```python
from build123d import *

# Parameters (mm, degrees)
SKETCH1_R           = 3.5875
SKETCH1_R_2         = 1.5875
BOSS_EXTRUDE1_DEPTH = 10
SKETCH2_R           = 1.5875
BOSS_EXTRUDE2_DEPTH = 10
BOSS_EXTRUDE3_REACH = 7.279


with BuildPart() as part:
    # Sketch1 → Boss-Extrude1 (new body)
    with BuildSketch(Plane.XY):
        Circle(SKETCH1_R)
        Circle(SKETCH1_R_2, mode=Mode.SUBTRACT)
    extrude(amount=BOSS_EXTRUDE1_DEPTH)

    # Sketch2 → Boss-Extrude2 (add)
    with BuildSketch(Plane(origin=(0, -1.69195383, 0), x_dir=(1, 0, 0), z_dir=(0, 1, 0))):
        with BuildLine():
            Line((-3.5875, -5), (-3.5875, -10))
            Line((-3.5875, -10), (3.5875, -10))
            Line((3.5875, -10), (3.5875, -5))
            ThreePointArc((3.5875, -5), (0, -1.4125), (-3.5875, -5))
        make_face()
        with Locations((0, -5)):
            Circle(SKETCH2_R, mode=Mode.SUBTRACT)
    extrude(amount=-BOSS_EXTRUDE2_DEPTH)

    # Sketch3 → Boss-Extrude3 (add, up to next)
    with BuildSketch(Plane(origin=(0, -1.69195383, 0), x_dir=(1, 0, 0), z_dir=(0, 1, 0)), mode=Mode.PRIVATE) as boss_extrude3_sk1:
        with BuildLine():
            Line((-3.5875, -10), (-3.5875, -5))
            ThreePointArc((-3.5875, -5), (-3.479874394, -4.127858699), (-3.16345515, -3.30804617))
            Line((-3.16345515, -3.30804617), (-3.16345515, -10))
            Line((-3.16345515, -10), (-3.5875, -10))
        make_face()
    boss_extrude3_tool1 = extrude(boss_extrude3_sk1.sketch, amount=BOSS_EXTRUDE3_REACH, mode=Mode.PRIVATE) - part.part
    add(boss_extrude3_tool1.solids().sort_by_distance((-3.367759, -1.691954, 6.916202))[0])
    # Sketch3 → Boss-Extrude3 (add, up to next)
    with BuildSketch(Plane(origin=(0, -1.69195383, 0), x_dir=(1, 0, 0), z_dir=(0, 1, 0)), mode=Mode.PRIVATE) as boss_extrude3_sk2:
        with BuildLine():
            Line((3.16345515, -10), (3.16345515, -3.30804617))
            ThreePointArc((3.16345515, -3.30804617), (3.479874394, -4.127858699), (3.5875, -5))
            Line((3.5875, -5), (3.5875, -10))
            Line((3.5875, -10), (3.16345515, -10))
        make_face()
    boss_extrude3_tool2 = extrude(boss_extrude3_sk2.sketch, amount=BOSS_EXTRUDE3_REACH, mode=Mode.PRIVATE) - part.part
    add(boss_extrude3_tool2.solids().sort_by_distance((3.367759, -1.691954, 6.916202))[0])


solid = part.part
```
Source: CAD feature listing. Evaluate the final solid. Frame: model axes, mm. A direction names the side the tool comes from. Coordinates: 2 decimals unless noted, no trailing zeros. Write each loop counter-clockwise with the first axis right and the second up, starting at its lowest first coordinate (ties: lowest second). Pieces come first, ordered by that corner, then holes. Notation, with made-up numbers: M -25,78.25 L 32,78.25 A23 ccw 32,87.25 Z; hole C 77.25,-9 d9. An arc over 180 degrees is marked long. Answer as a JSON object with one key per item and string values.
1. Draft query along X for faces 1 (the cylindrical face through (-0.023, -3.587, 4.978)), 2 (the flat face through (2, -1, 0)), 3 (the flat face through (3.588, -6, 7)). Return one class per face: released by +X, released by -X, zero draft, split by the parting line, or undercut.
Evaluation:
{"face 1": "undercut", "face 2": "zero draft", "face 3": "released by +X"}
2. Cut plane A-A on x = 0. Output: boundary loops of the cut face in (y, z), plus the area to 3 significant figures.
Evaluation:
{"outline": "M -11.69,1.41 L -3.59,1.41 L -3.59,0 L -1.59,0 L -1.59,10 L -11.69,10 L -11.69,6.59 L -3.59,6.59 L -3.59,3.41 L -11.69,3.41 Z; M 1.59,0 L 3.59,0 L 3.59,10 L 1.59,10 Z", "area": "83.9 mm^2"}
3. Contact query for flat-ended pins moving along their axis: P1, Ø1, axis at x = 2, z = 4, coming from the +Y side; P2, Ø3, axis at x = 0, z = 5, coming from the -Y side. Output: stop coordinate, or through.
Evaluation:
{"P1": "y = 3.26", "P2": "y = -3.59"}
4. Cut plane C-C on y = 0.5. Output: boundary loops of the cut face in (x, z), plus the area to 3 significant figures.
Evaluation:
{"outline": "M -3.55,0 L -1.51,0 L -1.51,10 L -3.55,10 Z; M 1.51,0 L 3.55,0 L 3.55,10 L 1.51,10 Z", "area": "40.9 mm^2"}
5. Ray query, L1, parallel to Z at x = 0, y = -5.5; L2, parallel to X at y = -8, z = 5. Return the intervals inside material, ascending.
Evaluation:
{"L1": "1.41 to 3.41, 6.59 to 10", "L2": "-3.59 to -1.59, 1.59 to 3.59"}
6. Access query for faces 4 (the cylindrical face through (-0.34, -7.4, 6.55)), 5 (the flat face through (0, -4, 10)), 6 (the cylindrical face through (-0.467, 3.557, 3.819)). Directions: +Z, -Z, +X, -X, +Y, -Y. A direction counts if a zero-diameter tool reaches every point of the face in a straight line with its end or side. Return the directions, or none.
Evaluation:
{"face 4": "-Y", "face 5": "+Z, +X, -X, +Y, -Y", "face 6": "-Z"}
7. Cut plane B-B on z = 7.25. Output: boundary loops of the cut face in (x, y) (1 decimal), plus the area to 3 significant figures.
Evaluation:
{"outline": "M -3.6,-11.7 L 3.6,-11.7 L 3.6,0 A3.6 ccw -3.6,0 Z; hole C 0,0 d3.2", "area": "96.2 mm^2"}
